```python
from build123d import *

# Parameters (mm, degrees)
F1_W     = 40
F1_H     = 73.52
F2_DEPTH = 10
F3_DEPTH = 4
F4_SIZE  = 3
F5_SIZE  = 3
F6_W     = 4
F6_H     = 48
F7_DEPTH = 25
F8_SIZE  = 3.99999


# Not quite as in the source:
# - a fillet or chamfer is up to 0.001 mm smaller than in the source, because OpenCascade refuses the exact size


with BuildPart() as f2:
    # F1 (on Front) → F2 (new body)
    with BuildSketch(Plane.XZ):
        Rectangle(F1_W, F1_H)
    extrude(amount=F2_DEPTH)

    # F0 (on Front) → F3 (cut)
    with BuildSketch(Plane.XZ):
        Polygon((2.3094010768, 4), (-2.3094010768, 4), (-4.6188021535, 0), (-2.3094010768, -4), (2.3094010768, -4), (4.6188021535, 0), align=None)
        Polygon((2.3094010768, 32), (-2.3094010768, 32), (-4.6188021535, 28), (-2.3094010768, 24), (2.3094010768, 24), (4.6188021535, 28), align=None)
        Polygon((2.3094010768, -24), (-2.3094010768, -24), (-4.6188021535, -28), (-2.3094010768, -32), (2.3094010768, -32), (4.6188021535, -28), align=None)
    extrude(amount=F3_DEPTH, mode=Mode.SUBTRACT)

    # F4
    f4_edges = [f2.edges().sort_by_distance(p)[0] for p in [
        (20, -5, -36.76),
    ]]
    chamfer(f4_edges, length=F4_SIZE)

    # F5
    f5_edges = [f2.edges().sort_by_distance(p)[0] for p in [
        (-20, -5, -36.76),
    ]]
    chamfer(f5_edges, length=F5_SIZE)

    # F6 (on Front) → F7 (cut)
    with BuildSketch(Plane.XZ):
        with Locations((-18, 0)):
            Rectangle(F6_W, F6_H)
    extrude(amount=F7_DEPTH, mode=Mode.SUBTRACT)

    # F8 (size 4 in the source; OpenCascade refuses exactly that, so slightly less here)
    f8_edges = [f2.edges().sort_by_distance(p)[0] for p in [
        (-20, -5, 24),
        (-20, -5, -24),
    ]]
    chamfer(f8_edges, length=F8_SIZE)


solid = f2.part
```
For this review, take the finished solid that the model builds, in its own axes (mm). A direction names the side the tool comes from. Round coordinates to 2 decimals unless told otherwise and drop trailing zeros. Write each loop counter-clockwise with the first axis right and the second up, starting at its lowest first coordinate (ties: lowest second). Pieces come first, ordered by that corner, then holes. Notation, with made-up numbers: (65.5, -37) -> (88.5, -37) arc R23 cw to (88.5, -13) -> close; hole circle Ø7 at (9, 37). An arc over 180 degrees is marked (long way). One line per question, with ' | ' between items. Start each with the question number.
(1) Add section A-A, the plane y = -2. Give the number of separate pieces and of enclosed holes in the cut face, plus the area to 3 significant figures.
(2) Add section C-C, the plane z = 3. Write out the cut boundary in (x, y), plus the area to 3 significant figures.
(3) Mouldability with a two-part tool opening along Z and no side actions: class faces 4 (the face through (-3.448, -1.972, 2.028)), 5 (the face through (0, -10, 1)), 6 (the face through (0, -5, -36.76)) as released by +Z, released by -Z, zero draft, split by the parting line, or undercut.
(4) Insertion check: P1, Ø5, axis at x = 7.5, z = 18.5, coming from the +Y side; P2, Ø5, axis at y = -3, z = -2.5, coming from the -X side; P3, Ø2.5, axis at x = 0, z = -0.5, coming from the +Y side. Each pin has a flat end and moves straight along its axis. Give the tip position at first contact, or say it passes through.
(5) Add section D-D, the plane z = 30.5. Write out the cut boundary in (x, y).
(6) For line 1 along Z through (x, y) = (-0.5, -2.25); line 2 along X through (y, z) = (-1.5, 6); line 3 along Z through (x, y) = (-16.5, -2), list the stretches that pass through material, from the lowest coordinate up. Write a range as from..to.
(7) Tool access review of faces 1 (the face through (-18, -5, 26)), 2 (the face through (0, -2, -32)), 3 (the face through (-5, 0, 1)): name each direction out of +Z, -Z, +X, -X, +Y, -Y from which nothing blocks a thin tool from reaching the whole face with its end or side.
Answer list:
1) separate pieces: 1 | enclosed holes: 3 | area: 2,560 mm²
2) outline: (-16, -10) -> (20, -10) -> (20, 0) -> (2.89, 0) -> (2.89, -4) -> (-2.89, -4) -> (-2.89, 0) -> (-16, 0) -> close | area: 337 mm²
3) face 4: undercut | face 5: zero draft | face 6: released by -Z
4) P1: y = 0 | P2: x = -16 | P3: y = -4
5) outline: (-20, -10) -> (20, -10) -> (20, 0) -> (3.18, 0) -> (3.18, -4) -> (-3.18, -4) -> (-3.18, 0) -> (-20, 0) -> close
6) line 1: -36.76..-32, -24..-4, 4..24, 32..36.76 | line 2: -16..20 | line 3: -36.76..-24.5, 24.5..36.76
7) face 1: -X, +Y, -Y | face 2: +Y | face 3: +Z, -Z, +X, -X, +Y
